CAD build for the part. Positions are in the model's coordinates, mm. Face numbers are marked on the shaded views. A direction names the side the tool comes from. Coordinates: 2 decimals unless noted, no trailing zeros. Loops run counter-clockwise (first coordinate to the right, second up) from the corner with the lowest first, then second, coordinate; pieces in that order, holes last. Notation, with made-up numbers: (83.5, -14.75) -> (118.5, -14.75) arc R21 cw to (118.5, 7.25) -> close; hole circle Ø7 at (79, 24.5). An arc over 180 degrees is marked (long way). Return JSON: item names as keys, results as strings. Group by question number.
(1) Flat gauge pins, fed straight in: pin 1 Ø1.3 at (y, z) = (-2.5, -2.5) entering from -X; pin 2 Ø5 at (y, z) = (7.5, 0.5) entering from +X; pin 3 Ø10 at (x, y) = (3, 9) entering from +Z. Where does each tip first touch, or does it go through?
(2) Saw through at C-C on z = -2.5. Write the cut outline in (x, y).
(3) Mould opens along Y. For the marked faces 1, 2, 3 and 4 say: pulls with the +Y half, pulls with the -Y half, needs draft (parallel to the pull), parting line crosses it, or undercut.
(4) Tool access for the marked faces 5, 6 and 7: list every direction of +Z, -Z, +X, -X, +Y, -Y with a clear straight run to the whole face (end or side of a thin tool).
(5) Saw through at A-A on z = 0.75. Write the cut outline in (x, y).
(6) Saw through at B-B on z = 6.5. Write the cut outline in (x, y), then the cut area to 3 significant figures.
(7) Probe L1, parallel to Y at x = 0, z = 0.6 (3 decimals); L2, parallel to Y at x = 0, z = 0.5 (3 decimals); L3, parallel to Z at x = -5, y = 8.25. List the from-to ranges inside material, lowest first.
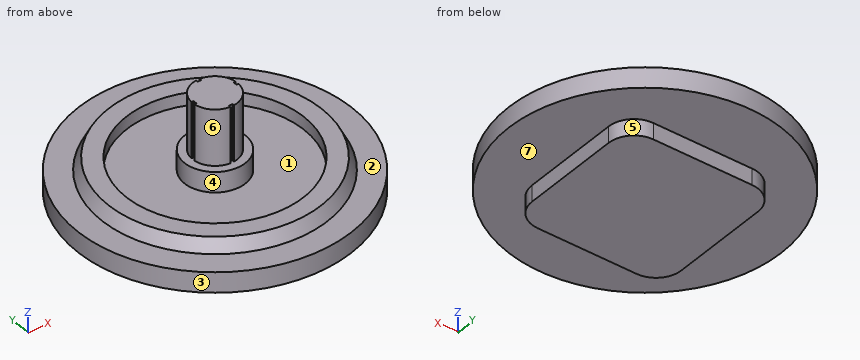
```python
from build123d import *

# Parameters (mm, degrees)
F0_R      = 13.5
F0_R_2    = 11.25
F0_R_3    = 10.5
F0_R_4    = 8.75
F0_R_5    = 3
F0_R_6    = 2.2
F1_DEPTH  = 2
F4_DEPTH  = 1.25
F6_DEPTH  = 2
F7_DEPTH  = 2
F8_DEPTH  = 6.25
F11_DEPTH = 1.6


# Not quite as in the source:
# - a fillet or chamfer that OpenCascade refuses, or shapes differently, is made with other operations: its cross-section is extruded or revolved along the edge and cut away or added


with BuildPart() as f1:
    # F0 (on Top) → F1 (new body)
    with BuildSketch(Plane.XY):
        Circle(F0_R)
        Circle(F0_R_2, mode=Mode.SUBTRACT)
        Circle(F0_R_2)
        Circle(F0_R_3, mode=Mode.SUBTRACT)
        Circle(F0_R_3)
        Circle(F0_R_4, mode=Mode.SUBTRACT)
        Circle(F0_R_4)
        Circle(F0_R_5, mode=Mode.SUBTRACT)
        Circle(F0_R_5)
        Circle(F0_R_6, mode=Mode.SUBTRACT)
        Circle(F0_R_6)
    extrude(amount=-F1_DEPTH)

    # F0 (on Top) → F4 (join)
    with BuildSketch(Plane.XY):
        Circle(F0_R_2)
        Circle(F0_R_3, mode=Mode.SUBTRACT)
        Circle(F0_R_3)
        Circle(F0_R_4, mode=Mode.SUBTRACT)
    extrude(amount=F4_DEPTH)

    # F5: chamfer of 1.5 x 0.75 on 1 edges, made by hand


with BuildPart() as f5_tool2:
    # F5_s3 → F5_t4 (revolve)
    with BuildSketch(Plane.XZ):
        Polygon((11.25, -0.25), (10.5, 1.25), (11.25, 1.25), align=None)
    revolve(axis=Axis((0, 0, 1.25), (0, 0, 1)))

    split(bisect_by=Plane.XY, keep=Keep.TOP)


with BuildPart() as f1_1:
    add(f1.part)

    # F5_t1: cut F5_tool2
    add(f5_tool2.part, mode=Mode.SUBTRACT)

    # F0 (on Top) → F6 (join)
    with BuildSketch(Plane.XY):
        Circle(F0_R_5)
        Circle(F0_R_6, mode=Mode.SUBTRACT)
    extrude(amount=F6_DEPTH)

    # F0 (on Top) → F7 (join)
    with BuildSketch(Plane.XY):
        Circle(F0_R_6)
    extrude(amount=F7_DEPTH)

    # F3 (on offset) → F8 (join)
    with BuildSketch(Plane.XY.offset(1.25)):
        with BuildLine():
            Line((-0.1818181818, 1.9917183909), (-0.1833333333, 2.1923478029))
            ThreePointArc((-0.1833333333, 2.1923478029), (-1.5556349186, 1.5556349186), (-2.1923478029, 0.1833333333))
            Line((-2.1923478029, 0.1833333333), (-1.9917183909, 0.1818181818))
            ThreePointArc((-1.9917183909, 0.1818181818), (-2, 0), (-1.9917183909, -0.1818181818))
            Line((-1.9917183909, -0.1818181818), (-2.1923478029, -0.1833333333))
            ThreePointArc((-2.1923478029, -0.1833333333), (-1.5556349186, -1.5556349186), (-0.1833333333, -2.1923478029))
            Line((-0.1833333333, -2.1923478029), (-0.1818181818, -1.9917183909))
            ThreePointArc((-0.1818181818, -1.9917183909), (0, -2), (0.1818181818, -1.9917183909))
            Line((0.1818181818, -1.9917183909), (0.1833333333, -2.1923478029))
            ThreePointArc((0.1833333333, -2.1923478029), (1.5556349186, -1.5556349186), (2.1923478029, -0.1833333333))
            Line((2.1923478029, -0.1833333333), (1.9917183909, -0.1818181818))
            ThreePointArc((1.9917183909, -0.1818181818), (2, 0), (1.9917183909, 0.1818181818))
            Line((1.9917183909, 0.1818181818), (2.1923478029, 0.1833333333))
            ThreePointArc((2.1923478029, 0.1833333333), (1.5556349186, 1.5556349186), (0.1833333333, 2.1923478029))
            Line((0.1833333333, 2.1923478029), (0.1818181818, 1.9917183909))
            ThreePointArc((0.1818181818, 1.9917183909), (0, 2), (-0.1818181818, 1.9917183909))
        make_face()
    extrude(amount=F8_DEPTH)

    # F10 (on offset) → F11 (join)
    with BuildSketch(Plane(origin=(0, 0, -2), x_dir=(1, 0, 0), z_dir=(0, 0, -1))):
        with BuildLine():
            Line((-4.9, -7.4), (4.9, -7.4))
            ThreePointArc((4.9, -7.4), (6.667766953, -6.667766953), (7.4, -4.9))
            Line((7.4, -4.9), (7.4, 4.9))
            ThreePointArc((7.4, 4.9), (6.667766953, 6.667766953), (4.9, 7.4))
            Line((4.9, 7.4), (-4.9, 7.4))
            ThreePointArc((-4.9, 7.4), (-6.667766953, 6.667766953), (-7.4, 4.9))
            Line((-7.4, 4.9), (-7.4, -4.9))
            ThreePointArc((-7.4, -4.9), (-6.667766953, -6.667766953), (-4.9, -7.4))
        make_face()
    extrude(amount=F11_DEPTH)


solid = f1_1.part
```
Geometry results:
{
 "1": {"pin 1": "x = -13.34", "pin 2": "x = 12.52", "pin 3": "z = 1.25"},
 "2": {"outline": "(-7.4, -4.9) arc R2.5 ccw to (-4.9, -7.4) -> (4.9, -7.4) arc R2.5 ccw to (7.4, -4.9) -> (7.4, 4.9) arc R2.5 ccw to (4.9, 7.4) -> (-4.9, 7.4) arc R2.5 ccw to (-7.4, 4.9) -> close"},
 "3": {"face 1": "undercut", "face 2": "needs draft", "face 3": "parting line crosses it", "face 4": "undercut"},
 "4": {"face 5": "-Z, +X, +Y", "face 6": "+Z, -X, -Y", "face 7": "-Z"},
 "5": {"outline": "circle Ø21.5 at (0, 0); circle Ø6 at (0, 0); hole circle Ø17.5 at (0, 0)"},
 "6": {"outline": "(-2.19, -0.18) arc R2.2 ccw to (-0.18, -2.19) -> (-0.18, -1.99) arc R2 ccw to (0.18, -1.99) -> (0.18, -2.19) arc R2.2 ccw to (2.19, -0.18) -> (1.99, -0.18) arc R2 ccw to (1.99, 0.18) -> (2.19, 0.18) arc R2.2 ccw to (0.18, 2.19) -> (0.18, 1.99) arc R2 ccw to (-0.18, 1.99) -> (-0.18, 2.19) arc R2.2 ccw to (-2.19, 0.18) -> (-1.99, 0.18) arc R2 ccw to (-1.99, -0.18) -> close", "area": "14.9 mm²"},
 "7": {"L1": "-10.825 to -8.75, -3 to 3, 8.75 to 10.825", "L2": "-10.875 to -8.75, -3 to 3, 8.75 to 10.875", "L3": "-2 to 1.25"}
}
